from build123d import *

# Parameters (mm, degrees)
SKETCH4_W            = 31.4
SKETCH4_H            = 31.4
SKETCH4_W_2          = 25.4
SKETCH4_H_2          = 25.4
BOSS_EXTRUDE3_DEPTH  = 30
SKETCH5_W            = 31.4
SKETCH5_H            = 31.4
BOSS_EXTRUDE4_DEPTH  = 5
SKETCH6_W            = 31.4
SKETCH6_H            = 8
BOSS_EXTRUDE5_DEPTH  = 5
BOSS_EXTRUDE6_DEPTH  = 8
SKETCH8_R            = 9.5
BOSS_EXTRUDE7_DEPTH  = 8
SKETCH9_W            = 31.4
SKETCH9_H            = 10
BOSS_EXTRUDE8_DEPTH  = 5
SKETCH10_W           = 31.4
SKETCH10_H           = 10
BOSS_EXTRUDE9_DEPTH  = 13
SKETCH11_W           = 6.2
SKETCH11_H           = 10
BOSS_EXTRUDE10_DEPTH = 40
BOSS_EXTRUDE11_DEPTH = 3
CUT_EXTRUDE1_START   = 8
SKETCH8_2_R          = 9.5
CUT_EXTRUDE1_DEPTH   = 24


with BuildPart() as part:
    # Sketch4 → Boss-Extrude3 (new body)
    with BuildSketch(Plane.XY):
        Rectangle(SKETCH4_W, SKETCH4_H)
        Rectangle(SKETCH4_W_2, SKETCH4_H_2, mode=Mode.SUBTRACT)
    extrude(amount=BOSS_EXTRUDE3_DEPTH)

    # Sketch5 → Boss-Extrude4 (add)
    with BuildSketch(Plane.XY.offset(30)):
        Rectangle(SKETCH5_W, SKETCH5_H)
    extrude(amount=BOSS_EXTRUDE4_DEPTH)

    # Sketch6 → Boss-Extrude5 (add)
    with BuildSketch(Plane.XY.offset(35)):
        Rectangle(SKETCH6_W, SKETCH6_H)
    extrude(amount=BOSS_EXTRUDE5_DEPTH)

    # Sketch7 → Boss-Extrude6 (add)
    with BuildSketch(Plane.XZ.offset(4)):
        with BuildLine():
            Line((-15.7, 40), (-15.7, 52))
            ThreePointArc((-15.7, 52), (-11.306601718, 62.606601718), (-0.7, 67))
            Line((-0.7, 67), (0.7, 67))
            ThreePointArc((0.7, 67), (11.306601718, 62.606601718), (15.7, 52))
            Line((15.7, 52), (15.7, 40))
            Line((15.7, 40), (-15.7, 40))
        make_face()
    extrude(amount=-BOSS_EXTRUDE6_DEPTH)

    # Sketch8 → Boss-Extrude7 (add)
    with BuildSketch(Plane.XZ.offset(4)):
        with Locations(Location((0, 52, 0), (0, 0, 180))):
            Circle(SKETCH8_R)
    boss_extrude7 = extrude(amount=BOSS_EXTRUDE7_DEPTH)

    # Mirror1: Boss-Extrude7 across plane
    add(boss_extrude7.mirror(Plane.ZX))

    # Sketch9 → Boss-Extrude8 (add)
    with BuildSketch(Plane(origin=(0, 15.7, 0), x_dir=(1, 0, 0), z_dir=(0, 1, 0))):
        with Locations((0, -27)):
            Rectangle(SKETCH9_W, SKETCH9_H)
    extrude(amount=BOSS_EXTRUDE8_DEPTH)

    # Sketch10 → Boss-Extrude9 (add)
    with BuildSketch(Plane(origin=(0, 15.7, 0), x_dir=(1, 0, 0), z_dir=(0, 1, 0))):
        with Locations((0, -17)):
            Rectangle(SKETCH10_W, SKETCH10_H)
    extrude(amount=BOSS_EXTRUDE9_DEPTH)

    # Sketch11 → Boss-Extrude10 (add)
    with BuildSketch(Plane(origin=(0, 20.7, 0), x_dir=(1, 0, 0), z_dir=(0, 1, 0))):
        with Locations((-12.6, -27)):
            Rectangle(SKETCH11_W, SKETCH11_H)
        with Locations((12.6, -27)):
            Rectangle(SKETCH11_W, SKETCH11_H)
    extrude(amount=BOSS_EXTRUDE10_DEPTH)

    # Sketch12 → Boss-Extrude11 (add)
    with BuildSketch(Plane.XY.offset(32)):
        Polygon((-15.7, 60.7), (-9.5, 60.7), (-9.5, 20.7), (9.5, 20.7), (9.5, 60.7), (15.7, 60.7), (15.7, 15.7), (-15.7, 15.7), align=None)
    extrude(amount=BOSS_EXTRUDE11_DEPTH)

    # Sketch8_2 → Cut-Extrude1 (cut)
    with BuildSketch(Plane.XZ.offset(4).offset(CUT_EXTRUDE1_START)):
        with Locations(Location((0, 52, 0), (0, 0, 270))):
            Circle(SKETCH8_2_R)
    extrude(amount=-CUT_EXTRUDE1_DEPTH, mode=Mode.SUBTRACT)


solid = part.part
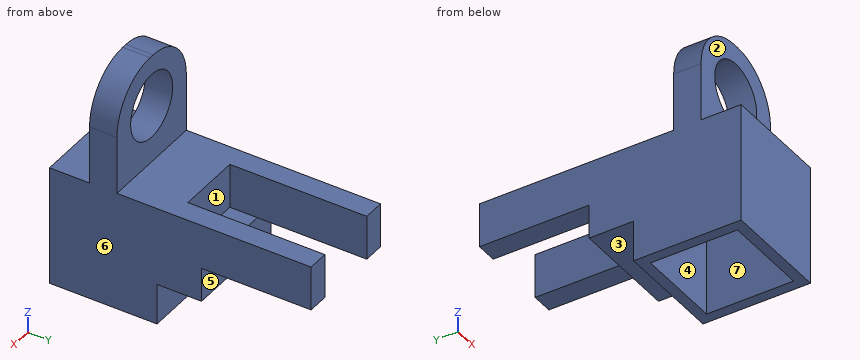
Can you work these out from the model? Positions are in its coordinate system, mm. Face numbers are marked on the shaded views. A direction names the side the tool comes from. Round coordinates to 2 decimals unless told otherwise and drop trailing zeros. Write each loop counter-clockwise with the first axis right and the second up, starting at its lowest first coordinate (ties: lowest second). Pieces come first, ordered by that corner, then holes. Notation, with made-up numbers: (10, 22.5) -> (61, 22.5) arc R19 ccw to (61, 41.5) -> close; hole circle Ø3 at (79.5, -14.75). An arc over 180 degrees is marked (long way). One line per question, with ' | ' between items. Start each with the question number.
1) Suppose I cut it at D-D on y = 25.5. Write out the boundary of the cut face in (x, z), then the cut area to 3 significant figures.
2) If we mould it in two halves opening along X, with no side actions, what happens to the marked faces 4, 5, 6 and 7? For each: released by +X, released by -X, zero draft, split by the parting line, or undercut.
3) Suppose I cut it at B-B on z = 47. Write out the boundary of the cut face in (x, y), then the cut area to 3 significant figures.
4) Suppose I cut it at C-C on x = -7.5. Write out the boundary of the cut face in (y, z).
5) I need wall thicknesses on line 1 (Y direction, x = 10, z = 3); line 2 (X direction, y = 0, z = 52). Which ranges of each line are inside material? Lowest first, please. Write a range as [from, to].
6) Suppose I cut it at A-A on y = 41. Write out the boundary of the cut face in (x, z), then the cut area to 3 significant figures.
7) I'm going to push flat-ended pins straight in: P1, Ø1.5, axis at x = 3.5, y = -7, coming from the -Z side; P2, Ø9.5, axis at x = 5, z = 8.5, coming from the +Y side; P3, Ø15.5, axis at x = 7, y = 26.5, coming from the +Z side; P4, Ø17, axis at x = 0, z = 52, coming from the +Y side. Where does each tip first touch, or does it pass through?
8) On a 3-axis mill with a long thin cutter (end or side, diameter ignored), from which of +Z, -Z, +X, -X, +Y, -Y can I reach the whole of each face in a straight line? I mean the marked faces 1, 2 and 3. Say none if no direction works.
Return value:
1) outline: (-15.7, 12) -> (15.7, 12) -> (15.7, 35) -> (9.5, 35) -> (9.5, 22) -> (-9.5, 22) -> (-9.5, 35) -> (-15.7, 35) -> close | area: 475 mm2
2) face 4: undercut | face 5: zero draft | face 6: released by +X | face 7: undercut
3) outline: (-15.7, -4) -> (-8.08, -4) -> (-8.08, 4) -> (-15.7, 4) -> close; (8.08, -4) -> (15.7, -4) -> (15.7, 4) -> (8.08, 4) -> close | area: 122 mm2
4) outline: (-15.7, 0) -> (-12.7, 0) -> (-12.7, 30) -> (12.7, 30) -> (12.7, 0) -> (15.7, 0) -> (15.7, 12) -> (28.7, 12) -> (28.7, 22) -> (20.7, 22) -> (20.7, 35) -> (4, 35) -> (4, 46.17) -> (-4, 46.17) -> (-4, 35) -> (-15.7, 35) -> close; (-4, 57.83) -> (4, 57.83) -> (4, 65.37) -> (-4, 65.37) -> close
5) line 1: y = [-15.7, -12.7], [12.7, 15.7] | line 2: x = [-15.7, -9.5], [9.5, 15.7]
6) outline: (-15.7, 22) -> (-9.5, 22) -> (-9.5, 35) -> (-15.7, 35) -> close; (9.5, 22) -> (15.7, 22) -> (15.7, 35) -> (9.5, 35) -> close | area: 161 mm2
7) P1: stops at z = 30 | P2: stops at y = 28.7 | P3: stops at z = 35 | P4: passes through
8) face 1: +Z, +Y | face 2: +Z, +X, -X, -Y | face 3: -Z, +X, -X, +Y
